Input: part model. Units: mm. Frame: model coordinates. Round coordinates to 2 decimals unless told otherwise and drop trailing zeros. Order: outer loops, then holes, each group sorted by start corner. A loop starts at its lowest first (then second) coordinate and runs counter-clockwise, first axis right, second up.
Item 1: Line query: L1, parallel to Y at x = 247.75, z = -48; L2, parallel to Y at x = 240.25, z = -9.5; L3, parallel to Y at x = 241.5, z = -3.5. Output: solid intervals per line, ascending.
Item 2: Mould query, pull axis Y, two halves, no side actions, for faces 1 (the cylindrical face through (243.593, 446.027, -57.824)), 2 (the flat face through (238.523, 446, -31)). Classes: released by +Y, released by -Y, zero draft, split by the parting line, or undercut.
Item 3: First-contact query: pin 1 (3 mm diameter, centred on x = 245, y = 876, fed in from +Z); pin 2 (0.7 mm diameter, centred on x = 245, z = -69.5, fed in from +Y); pin 3 (2 mm diameter, centred on x = 242.5, y = 346, fed in from -Z). Flat tips, straight axial feed; report the tip coordinate or a pass-through.
Item 4: Cut plane A-A on y = 698.5. Output: boundary loops of the cut face in (x, z).
Item 5: Cut plane B-B on x = 246.5. Give the number of separate pieces and of enclosed holes in the cut face, then the cut area to 3 significant figures.
Item 6: Cut plane C-C on y = 359. Output: boundary loops of the cut face in (x, z).
```python
from build123d import *

# Parameters (mm, degrees)
DODANIE_WYCI_GNI_CIE1_DEPTH = 10
SZKIC1_W                    = 30
SZKIC1_H                    = 10.1
SZKIC1_W_2                  = 25
WYTNIJ_WYCI_GNI_CIE1_DEPTH  = 10
WYTNIJ_WYCI_GNI_CIE2_DEPTH  = 10
SZYK_LINIOWY1_COUNT         = 2
SZYK_LINIOWY1_PITCH         = 55
SZKIC7_R                    = 2.45
WYTNIJ_WYCI_GNI_CIE5_DEPTH  = 10
SZYK_LINIOWY3_COUNT         = 6
SZYK_LINIOWY3_PITCH         = 100
SZKIC8_W                    = 13
SZKIC8_H                    = 22
WYTNIJ_WYCI_GNI_CIE6_DEPTH  = 10
LUSTRO1_COPY_1_DEPTH        = 10
SZKIC12_R                   = 1.55
WYTNIJ_WYCI_GNI_CIE7_DEPTH  = 10
SZYK_LINIOWY4_COUNT         = 2
SZYK_LINIOWY4_PITCH         = 223


with BuildPart() as part:
    # Szkic11 → Dodanie-wyciągnięcie1 (new body)
    with BuildSketch(Plane.ZY.offset(-248.52281754)):
        with BuildLine():
            Line((-79.001367167, 0), (0, 0))
            Line((0, 0), (0, 880))
            Line((0, 880), (-78.955177412, 880))
            Line((-78.955177412, 880), (-78.955177412, 870))
            ThreePointArc((-78.955177412, 870), (-57.819766969, 439.998863597), (-79.001367167, 10))
            Line((-79.001367167, 10), (-79.001367167, 0))
        make_face()
    extrude(amount=DODANIE_WYCI_GNI_CIE1_DEPTH)

    # Szkic1 → Wytnij-wyciągnięcie1 (cut)
    with BuildSketch(Plane(origin=(248.52281754, 0, 0), x_dir=(0, 0, -1), z_dir=(1, 0, 0))):
        with Locations((70, 874.95)):
            Rectangle(SZKIC1_W, SZKIC1_H)
        with Locations((12.5, 874.95)):
            Rectangle(SZKIC1_W_2, SZKIC1_H)
    wytnij_wyci_gni_cie1 = extrude(amount=-WYTNIJ_WYCI_GNI_CIE1_DEPTH, mode=Mode.SUBTRACT)

    # Szkic2 → Wytnij-wyciągnięcie2 (cut)
    with BuildSketch(Plane(origin=(248.52281754, 0, 0), x_dir=(0, 0, -1), z_dir=(1, 0, 0))):
        Polygon((10.660920663, 869.9), (13.760920663, 869.9), (13.760920663, 861.4), (15.135920663, 861.4), (15.135920663, 859.4), (13.760920663, 859.4), (13.760920663, 858.9), (10.660920663, 858.9), (10.660920663, 859.4), (9.285920663, 859.4), (9.285920663, 861.4), (10.660920663, 861.4), align=None)
    wytnij_wyci_gni_cie2 = extrude(amount=-WYTNIJ_WYCI_GNI_CIE2_DEPTH, mode=Mode.SUBTRACT)

    # Szyk liniowy1: Wytnij-wyciągnięcie2 ×2
    with Locations(*[(0, 0, -i * SZYK_LINIOWY1_PITCH) for i in range(1, SZYK_LINIOWY1_COUNT)]):
        add(wytnij_wyci_gni_cie2, mode=Mode.SUBTRACT)

    # Szkic7 → Wytnij-wyciągnięcie5 (cut)
    with BuildSketch(Plane(origin=(248.52281754, 0, 0), x_dir=(0, 0, -1), z_dir=(1, 0, 0))):
        with Locations((14.31069395, 742.236985413)):
            Circle(SZKIC7_R)
    wytnij_wyci_gni_cie5 = extrude(amount=-WYTNIJ_WYCI_GNI_CIE5_DEPTH, mode=Mode.SUBTRACT)

    # Szyk liniowy3: Wytnij-wyciągnięcie5 ×6
    with Locations(*[(0, -i * SZYK_LINIOWY3_PITCH, 0) for i in range(1, SZYK_LINIOWY3_COUNT)]):
        add(wytnij_wyci_gni_cie5, mode=Mode.SUBTRACT)

    # Szkic8 → Wytnij-wyciągnięcie6 (cut)
    with BuildSketch(Plane(origin=(248.52281754, 0, 0), x_dir=(0, 0, -1), z_dir=(1, 0, 0))):
        with Locations((6.5, 71)):
            Rectangle(SZKIC8_W, SZKIC8_H)
    extrude(amount=-WYTNIJ_WYCI_GNI_CIE6_DEPTH, mode=Mode.SUBTRACT)

    # Lustro1: Wytnij-wyciągnięcie1, Wytnij-wyciągnięcie2 across plane
    add(wytnij_wyci_gni_cie1.mirror(Plane.ZX.offset(440)), mode=Mode.SUBTRACT)
    add(wytnij_wyci_gni_cie2.mirror(Plane.ZX.offset(440)), mode=Mode.SUBTRACT)

    # Lustro1 copy 1 sketch → Lustro1 copy 1 (cut)
    with BuildSketch(Plane(origin=(248.52281754, 880, -55), x_dir=(0, 0, -1), z_dir=(1, 0, 0))):
        Polygon((10.660920663, -869.9), (13.760920663, -869.9), (13.760920663, -861.4), (15.135920663, -861.4), (15.135920663, -859.4), (13.760920663, -859.4), (13.760920663, -858.9), (10.660920663, -858.9), (10.660920663, -859.4), (9.285920663, -859.4), (9.285920663, -861.4), (10.660920663, -861.4), align=None)
    extrude(amount=-LUSTRO1_COPY_1_DEPTH, mode=Mode.SUBTRACT)

    # Szkic12 → Wytnij-wyciągnięcie7 (cut)
    with BuildSketch(Plane.ZY.offset(-238.52281754)):
        with Locations((-47.7, 380.736985413)):
            Circle(SZKIC12_R)
        with Locations((-16.7, 380.736985413)):
            Circle(SZKIC12_R)
    wytnij_wyci_gni_cie7 = extrude(amount=-WYTNIJ_WYCI_GNI_CIE7_DEPTH, mode=Mode.SUBTRACT)

    # Szyk liniowy4: Wytnij-wyciągnięcie7 ×2
    with Locations(*[(0, i * SZYK_LINIOWY4_PITCH, 0) for i in range(1, SZYK_LINIOWY4_COUNT)]):
        add(wytnij_wyci_gni_cie7, mode=Mode.SUBTRACT)


solid = part.part
```
From the geometry:
1. L1: y = 0 to 379.22, 382.26 to 602.22, 605.26 to 880
1. L2: y = 10.1 to 18.6, 20.6 to 60, 82 to 859.4, 861.4 to 869.9
1. L3: y = 10.1 to 60, 82 to 869.9
2. face 1: undercut
2. face 2: zero draft
3. pin 1: stops at z = -25
3. pin 2: stops at y = 869.9
3. pin 3: stops at z = -58.86
4. outline: (238.52, -65.44) - (248.52, -65.44) - (248.52, 0) - (238.52, 0) - close
5. separate pieces: 1
5. enclosed holes: 10
5. area: 55,800 mm2
6. outline: (238.52, -58.57) - (248.52, -58.57) - (248.52, 0) - (238.52, 0) - close
